For this review, take the finished solid that the model builds, in its own axes (mm). Face numbers are marked on the shaded views. Coordinates: 2 decimals unless noted, no trailing zeros. Write each loop counter-clockwise with the first axis right and the second up, starting at its lowest first coordinate (ties: lowest second). Pieces come first, ordered by that corner, then holes.
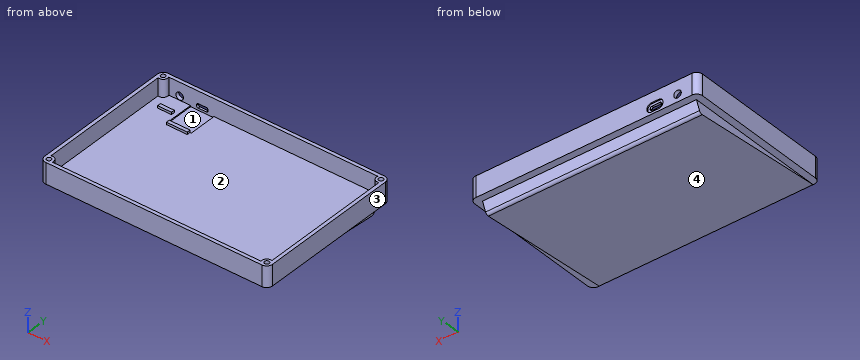
```python
from build123d import *

# Parameters (mm, degrees)
RIGHT_BODY_PAD_DEPTH            = 18
RIGHT_BODY_CAVITY_POCKET_DEPTH  = 15
RIGHT_BODY_BOSSES_R             = 4
RIGHT_BODY_BOSS_PAD_DEPTH       = 15
RIGHT_BODY_INSERT_HOLES_R       = 2
RIGHT_BODY_INSERT_POCKETS_DEPTH = 7
RIGHT_BODY_REST_PAD_DEPTH       = 92.343675
RIGHT_BODY_REST_FILLET_R        = 3
RIGHT_JACK_HOLE_R               = 3.25
RIGHT_JACK_HOLE_POCKET_DEPTH    = 3.2
RIGHT_JACK_STOP_W               = 12
RIGHT_JACK_STOP_H               = 3
RIGHT_JACK_STOP_PAD_DEPTH       = 2
OBJ1               = 20.2
OBJ2               = 24.2
OBJ3    = 1
RIGHT_USB_OPENING_POCKET_DEPTH  = 3.2
RIGHT_USB_BEZEL_POCKET_DEPTH    = 1.1
OBJ4               = 18
OBJ5               = 3
OBJ6       = 2


with BuildPart() as part:
    # Right_Body_Outline → Right_Body_Pad (new body)
    with BuildSketch(Plane.XY.offset(-18)):
        with BuildLine():
            Line((-0.38035, -5.791), (186.307, -5.791))
            ThreePointArc((186.307, -5.791), (189.842534, -4.326534), (191.307, -0.791))
            Line((191.307, -0.791), (191.307, 119.971))
            ThreePointArc((191.307, 119.971), (189.842534, 123.506534), (186.307, 124.971))
            Line((186.307, 124.971), (-0.38035, 124.971))
            ThreePointArc((-0.38035, 124.971), (-3.915884, 123.506534), (-5.38035, 119.971))
            Line((-5.38035, 119.971), (-5.38035, -0.791))
            ThreePointArc((-5.38035, -0.791), (-3.915884, -4.326534), (-0.38035, -5.791))
        make_face()
    extrude(amount=RIGHT_BODY_PAD_DEPTH)

    # Right_Body_Cavity → Right_Body_Cavity_Pocket (cut)
    with BuildSketch(Plane.XY):
        with BuildLine():
            Line((-0.38035, -2.791), (186.307, -2.791))
            ThreePointArc((186.307, -2.791), (187.721214, -2.205214), (188.307, -0.791))
            Line((188.307, -0.791), (188.307, 119.971))
            ThreePointArc((188.307, 119.971), (187.721214, 121.385214), (186.307, 121.971))
            Line((186.307, 121.971), (-0.38035, 121.971))
            ThreePointArc((-0.38035, 121.971), (-1.794564, 121.385214), (-2.38035, 119.971))
            Line((-2.38035, 119.971), (-2.38035, -0.791))
            ThreePointArc((-2.38035, -0.791), (-1.794564, -2.205214), (-0.38035, -2.791))
        make_face()
    extrude(amount=-RIGHT_BODY_CAVITY_POCKET_DEPTH, mode=Mode.SUBTRACT)

    # Right_Body_Bosses → Right_Body_Boss_Pad (join)
    with BuildSketch(Plane.XY.offset(-15)):
        with Locations((-1.08035, -1.491)):
            Circle(RIGHT_BODY_BOSSES_R)
        with Locations((187.007, -1.491)):
            Circle(RIGHT_BODY_BOSSES_R)
        with Locations((-1.08035, 120.671)):
            Circle(RIGHT_BODY_BOSSES_R)
        with Locations((187.007, 120.671)):
            Circle(RIGHT_BODY_BOSSES_R)
    extrude(amount=RIGHT_BODY_BOSS_PAD_DEPTH)

    # Right_Body_Insert_Holes → Right_Body_Insert_Pockets (cut)
    with BuildSketch(Plane.XY):
        with Locations((-1.08035, -1.491)):
            Circle(RIGHT_BODY_INSERT_HOLES_R)
        with Locations((187.007, -1.491)):
            Circle(RIGHT_BODY_INSERT_HOLES_R)
        with Locations((-1.08035, 120.671)):
            Circle(RIGHT_BODY_INSERT_HOLES_R)
        with Locations((187.007, 120.671)):
            Circle(RIGHT_BODY_INSERT_HOLES_R)
    extrude(amount=-RIGHT_BODY_INSERT_POCKETS_DEPTH, mode=Mode.SUBTRACT)

    # Right_Body_Rest → Right_Body_Rest_Pad (join, symmetric)
    with BuildSketch(Plane.YZ.offset(92.963325)):
        Polygon((-5.791, -18), (118.971, -18), (114.852748, -27.112629), align=None)
    extrude(amount=RIGHT_BODY_REST_PAD_DEPTH, both=True)

    # Right_Body_Rest_Fillet
    right_body_rest_fillet_edges = [part.edges().sort_by_distance(p)[0] for p in [
        (92.963325, 114.852748, -27.112629),
    ]]
    fillet(right_body_rest_fillet_edges, radius=RIGHT_BODY_REST_FILLET_R)

    # Right_Jack_Hole → Right_Jack_Hole_Pocket (cut)
    with BuildSketch(Plane.XZ.offset(-124.971)):
        with Locations((12.11965, -11.5)):
            Circle(RIGHT_JACK_HOLE_R)
    extrude(amount=RIGHT_JACK_HOLE_POCKET_DEPTH, mode=Mode.SUBTRACT)

    # Right_Jack_Stop → Right_Jack_Stop_Pad (join)
    with BuildSketch(Plane.XY.offset(-15)):
        with Locations((12.11965, 107.271)):
            Rectangle(RIGHT_JACK_STOP_W, RIGHT_JACK_STOP_H)
    extrude(amount=RIGHT_JACK_STOP_PAD_DEPTH)

    with BuildSketch(Plane.XY.offset(-15)):
        with Locations((31.62, 109.871)):
            Rectangle(OBJ1, OBJ2)
    extrude(amount=-OBJ3, mode=Mode.SUBTRACT)

    # Right_Usb_Opening → Right_Usb_Opening_Pocket (cut)
    with BuildSketch(Plane.XZ.offset(-124.971)):
        with BuildLine():
            Line((28.12, -14.15), (35.12, -14.15))
            ThreePointArc((35.12, -14.15), (36.18066, -13.71066), (36.62, -12.65))
            Line((36.62, -12.65), (36.62, -11.95))
            ThreePointArc((36.62, -11.95), (36.18066, -10.88934), (35.12, -10.45))
            Line((35.12, -10.45), (28.12, -10.45))
            ThreePointArc((28.12, -10.45), (27.05934, -10.88934), (26.62, -11.95))
            Line((26.62, -11.95), (26.62, -12.65))
            ThreePointArc((26.62, -12.65), (27.05934, -13.71066), (28.12, -14.15))
        make_face()
    extrude(amount=RIGHT_USB_OPENING_POCKET_DEPTH, mode=Mode.SUBTRACT)

    # Right_Usb_Bezel → Right_Usb_Bezel_Pocket (cut)
    with BuildSketch(Plane.XZ.offset(-124.971)):
        with BuildLine():
            Line((28.42, -16.15), (34.82, -16.15))
            ThreePointArc((34.82, -16.15), (37.507006, -15.037006), (38.62, -12.35))
            Line((38.62, -12.35), (38.62, -12.25))
            ThreePointArc((38.62, -12.25), (37.507006, -9.562994), (34.82, -8.45))
            Line((34.82, -8.45), (28.42, -8.45))
            ThreePointArc((28.42, -8.45), (25.732994, -9.562994), (24.62, -12.25))
            Line((24.62, -12.25), (24.62, -12.35))
            ThreePointArc((24.62, -12.35), (25.732994, -15.037006), (28.42, -16.15))
        make_face()
    extrude(amount=RIGHT_USB_BEZEL_POCKET_DEPTH, mode=Mode.SUBTRACT)

    with BuildSketch(Plane.XY.offset(-15)):
        with Locations((31.62, 96.271)):
            Rectangle(OBJ4, OBJ5)
    extrude(amount=OBJ6)


with BuildPart() as part_1:
    # Right_Keyboard_Body placement: moved
    add(part.part.moved(Location((174.06235, 0, 0))))


solid = part_1.part
```
Q1. Add section C-C (y = 22). State the section outline as (x, z) points, then the cut area to 3 significant figures.
Ans:
outline: (168.68, -18) - (174.68, -18) - (174.68, -20.1) - (359.37, -20.1) - (359.37, -18) - (365.37, -18) - (365.37, 0) - (362.37, 0) - (362.37, -15) - (171.68, -15) - (171.68, 0) - (168.68, 0) - close
area: 1,070 mm2
Q2. For probe 1 along X at (y, z) = (84.5, -14.25); probe 2 along Y at (x, z) = (328, -4.5); probe 3 along X at (y, z) = (123.25, -11.5), list the stretches that pass through material, from the lowest coordinate up.
Ans:
probe 1: x = 168.68 to 171.68, 362.37 to 365.37
probe 2: y = -5.79 to -2.79, 121.97 to 124.97
probe 3: x = 169.91 to 182.93, 189.43 to 200.75, 210.61 to 364.14
Q3. Add section D-D (y = 52.5). State the section outline as (x, z) points, then the cut area to 3 significant figures.
Ans:
outline: (168.68, -18) - (174.68, -18) - (174.68, -22.4) - (359.37, -22.4) - (359.37, -18) - (365.37, -18) - (365.37, 0) - (362.37, 0) - (362.37, -15) - (171.68, -15) - (171.68, 0) - (168.68, 0) - close
area: 1,490 mm2
Q4. Clearance check with flat-ended pins moving along their axes: pin 1 Ø6 at (x, y) = (201.5, 106) entering from +Z; pin 2 Ø3.5 at (x, y) = (187, 106.5) entering from +Z; pin 3 Ø1.2 at (x, y) = (172.5, 120.5) entering from +Z; pin 4 Ø6 at (x, z) = (204, -11) entering from +Y. State where each tip first meets the part, or that it passes through.
Ans:
pin 1: stops at z = -16
pin 2: stops at z = -13
pin 3: stops at z = -7
pin 4: stops at y = 124.97
Q5. Draft analysis for pull direction X (two halves, no side actions). For the marked faces 1, 2, 3 and 4, state which applies: +X half, -X half, draft (parallel to the pull), parting line (faces both ways), or undercut.
Ans:
face 1: undercut
face 2: undercut
face 3: +X half
face 4: draft
Q6. Add section A-A (x = 255.5). State the section outline as (y, z) points, then the cut area to 3 significant figures.
Ans:
outline: (-5.79, -18) - (112.76, -26.95) arc R3 ccw to (115.72, -25.2) - (118.97, -18) - (124.97, -18) - (124.97, 0) - (121.97, 0) - (121.97, -15) - (-2.79, -15) - (-2.79, 0) - (-5.79, 0) - close
area: 1,050 mm2
Q7. Add section B-B (z = -3.75). State the section outline as (x, y) points.
Ans:
outline: (168.68, -0.79) arc R5 ccw to (173.68, -5.79) - (360.37, -5.79) arc R5 ccw to (365.37, -0.79) - (365.37, 119.97) arc R5 ccw to (360.37, 124.97) - (173.68, 124.97) arc R5 ccw to (168.68, 119.97) - close; hole circle Ø4 at (172.98, -1.49); hole circle Ø4 at (172.98, 120.67); hole (171.68, 2.29) arc R4 cw to (176.76, -2.79) - (357.29, -2.79) arc R4 cw to (362.37, 2.29) - (362.37, 116.89) arc R4 cw to (357.29, 121.97) - (176.76, 121.97) arc R4 cw to (171.68, 116.89) - close; hole circle Ø4 at (361.07, -1.49); hole circle Ø4 at (361.07, 120.67)
